Source: CAD feature listing. Evaluate the final solid. Frame: model axes, mm. Coordinates: 2 decimals unless noted, no trailing zeros. Loops run counter-clockwise (first coordinate to the right, second up) from the corner with the lowest first, then second, coordinate; pieces in that order, holes last. Notation, with made-up numbers: (10, 16.25) -> (57, 16.25) arc R6 ccw to (57, 20.25) -> close; hole circle Ø5 at (-23.5, 46). An arc over 180 degrees is marked (long way). Answer as CSV lines item,"result".
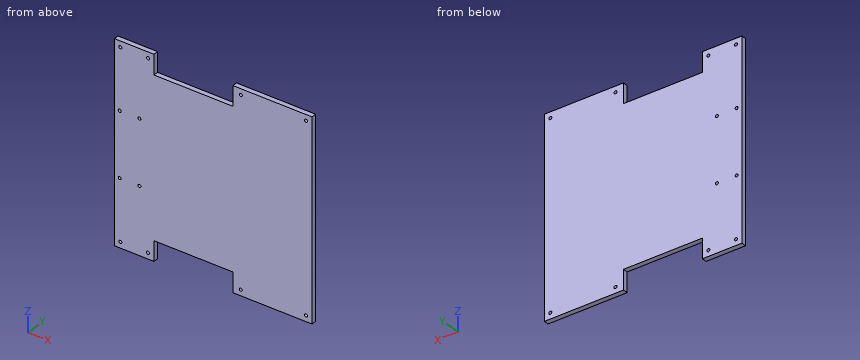
from build123d import *

# Parameters (mm, degrees)
BOSS_EXTRUDE1_DEPTH = 5
SKETCH2_R           = 1.5
CUT_EXTRUDE1_DEPTH  = 20
SKETCH3_R           = 1.5
CUT_EXTRUDE2_DEPTH  = 5


with BuildPart() as part:
    # Sketch1 → Boss-Extrude1 (new body)
    with BuildSketch(Plane(origin=(0, 0, 0), x_dir=(1, 0, 0), z_dir=(0, 1, 0))):
        Polygon((67.547169811, 149.902137597), (67.547169811, 129.902137597), (147.547169811, 129.902137597), (147.547169811, 149.902137597), (227.547169811, 149.902137597), (227.547169811, -50.097862403), (147.547169811, -50.097862403), (147.547169811, -30.097862403), (67.547169811, -30.097862403), (67.547169811, -50.097862403), (27.547169811, -50.097862403), (27.547169811, 149.902137597), align=None)
    extrude(amount=BOSS_EXTRUDE1_DEPTH)

    # Sketch2 → Cut-Extrude1 (cut)
    with BuildSketch(Plane(origin=(0, 5, 0), x_dir=(1, 0, 0), z_dir=(0, 1, 0))):
        with Locations(Location((33.547169811, 143.902137597, 0), (0, 0, 270))):
            Circle(SKETCH2_R)
        with Locations(Location((61.547169811, 143.902137597, 0), (0, 0, 270))):
            Circle(SKETCH2_R)
        with Locations(Location((33.547169811, -44.097862403, 0), (0, 0, 270))):
            Circle(SKETCH2_R)
        with Locations(Location((61.547169811, -44.097862403, 0), (0, 0, 270))):
            Circle(SKETCH2_R)
        with Locations(Location((155.547169811, -44.097862403, 0), (0, 0, 270))):
            Circle(SKETCH2_R)
        with Locations(Location((221.547169811, -44.097862403, 0), (0, 0, 270))):
            Circle(SKETCH2_R)
        with Locations(Location((155.547169811, 143.902137597, 0), (0, 0, 270))):
            Circle(SKETCH2_R)
        with Locations(Location((221.547169811, 143.902137597, 0), (0, 0, 270))):
            Circle(SKETCH2_R)
    extrude(amount=-CUT_EXTRUDE1_DEPTH, mode=Mode.SUBTRACT)

    # Sketch3 → Cut-Extrude2 (cut)
    with BuildSketch(Plane(origin=(0, 5, 0), x_dir=(1, 0, 0), z_dir=(0, 1, 0))):
        with Locations(Location((32.908431657, 82.511625863, 0), (0, 0, 270))):
            Circle(SKETCH3_R)
        with Locations(Location((32.908431657, 17.511625863, 0), (0, 0, 270))):
            Circle(SKETCH3_R)
        with Locations(Location((52.908431657, 17.511625863, 0), (0, 0, 270))):
            Circle(SKETCH3_R)
        with Locations(Location((52.908431657, 82.511625863, 0), (0, 0, 270))):
            Circle(SKETCH3_R)
    extrude(amount=-CUT_EXTRUDE2_DEPTH, mode=Mode.SUBTRACT)


solid = part.part
(1) Pin query (flat end, axial travel): pin 1 Ø2.5 at (x, y) = (100, 3) entering from -Z; pin 2 Ø1 at (x, y) = (78, 3) entering from +Z. Return the tip coordinate at first contact, or that it passes through.
Computed values:
pin 1,"z = -129.9"
pin 2,"z = 30.1"
(2) Cut plane B-B (y = 3.3). State how many separate pieces and enclosed holes the cut face has, then the cut area to 3 significant figures.
Computed values:
separate pieces,"1"
enclosed holes,"12"
area,"36,700 mm^2"
(3) Material intervals for L1, parallel to X at y = 3.1, z = 38; L2, parallel to X at y = 0.85, z = -16.5; L3, parallel to Z at x = 76.5, y = 4, sorted ascending. Write a range as [from, to].
Computed values:
L1,"[27.55, 67.55], [147.55, 227.55]"
L2,"[27.55, 31.8], [34.02, 51.8], [54.02, 227.55]"
L3,"[-129.9, 30.1]"
(4) Cut plane C-C (x = 144.5). Return the cut outline in (y, z).
Computed values:
outline,"(0, -129.9) -> (5, -129.9) -> (5, 30.1) -> (0, 30.1) -> close"
(5) Cut plane A-A (z = 32.5). Return the cut outline in (x, y).
Computed values:
outline,"(27.55, 0) -> (67.55, 0) -> (67.55, 5) -> (27.55, 5) -> close; (147.55, 0) -> (227.55, 0) -> (227.55, 5) -> (147.55, 5) -> close"
